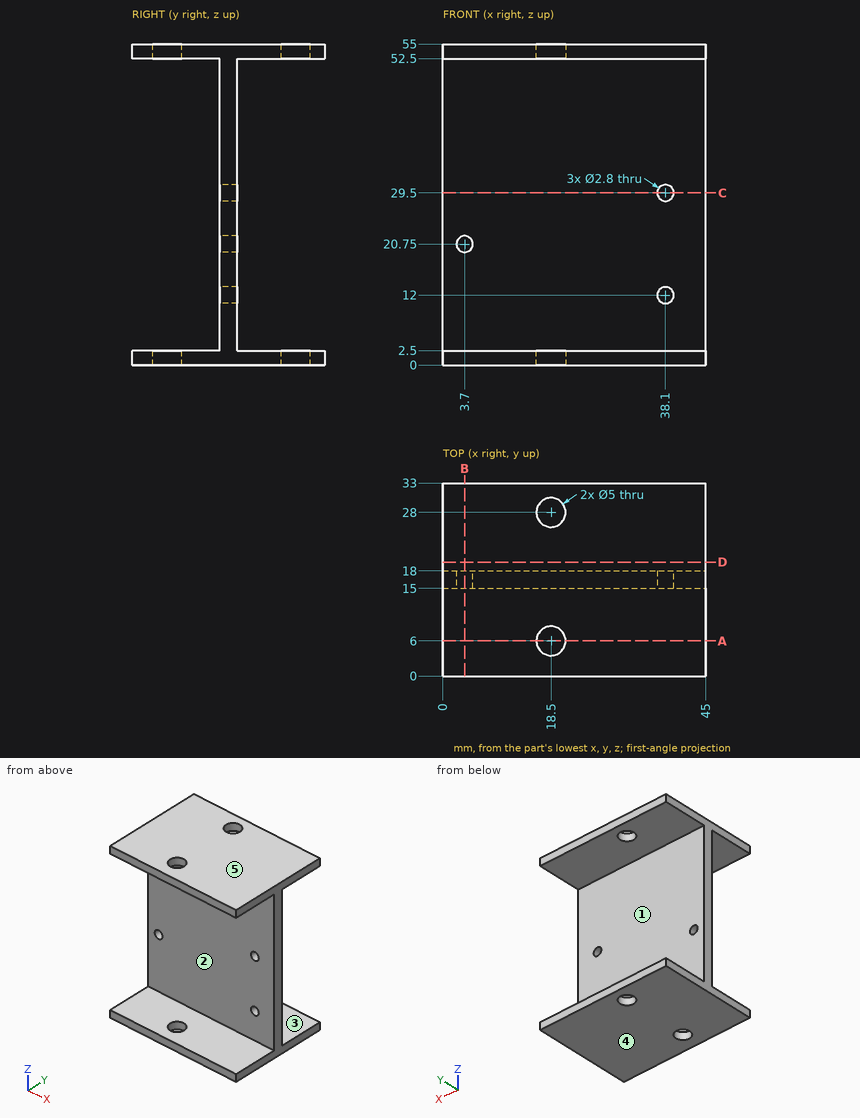
Verification items for this drawing (mm, ordinates from the low corner). A direction names the side the tool comes from. Give positions to 0.01 mm unless a question says otherwise; leave off trailing zeros. Write each loop counter-clockwise with the first axis right and the second up, starting at its lowest first coordinate (ties: lowest second). Pieces come first, ordered by that corner, then holes. Notation, with made-up numbers: (80.5, 72) -> (102.5, 72) arc R11 ccw to (102.5, 93) -> close; hole circle Ø2 at (20, -1.5). An arc over 180 degrees is marked (long way). Use CSV: the item, a comma, the result in double quotes. Start each with the question number.
Q1. Cross-section at A-A on y = 6. Enter the section's corners in (x, z).
Q2. Cross-section at B-B on x = 3.7. Enter the section's corners in (y, z).
Q3. Tool access check on the marked faces 1 and 2. Record the directions out of +Z, -Z, +X, -X, +Y, -Y that give a thin tool (end or side, any length) a straight path to the whole face; none if there is none.
Q4. Depth check by flat-ended pin: P1, Ø5, axis at x = 17, z = 31, coming from the +Y side; P2, Ø4.5, axis at x = 3.7, z = 20.75, coming from the -Y side. Enter the tip coordinate at first touch or a pass-through.
Q5. Cross-section at C-C on z = 29.5. Enter the section's corners in (x, y), and give its area (3 significant figures).
Q6. Release check for a two-part mould opening along Z. For the marked faces 3, 4 and 5 record: +Z half, -Z half, draft (parallel to the pull), parting line (faces both ways), or undercut.
Q7. Scan lines: line 1 along Y through (x, z) = (18.5, 54.55); line 2 along Z through (x, y) = (10, 5.5); line 3 along Z through (x, y) = (38.1, 15.95). Record each from-to range of solid material in increasing order.
Q8. Cross-section at D-D on y = 19.5. Enter the section's corners in (x, z).
Working result:
1,outline,"(0, 0) -> (16, 0) -> (16, 2.5) -> (0, 2.5) -> close; (0, 52.5) -> (16, 52.5) -> (16, 55) -> (0, 55) -> close; (21, 0) -> (45, 0) -> (45, 2.5) -> (21, 2.5) -> close; (21, 52.5) -> (45, 52.5) -> (45, 55) -> (21, 55) -> close"
2,outline,"(0, 0) -> (33, 0) -> (33, 2.5) -> (18, 2.5) -> (18, 19.35) -> (15, 19.35) -> (15, 2.5) -> (0, 2.5) -> close; (0, 52.5) -> (15, 52.5) -> (15, 22.15) -> (18, 22.15) -> (18, 52.5) -> (33, 52.5) -> (33, 55) -> (0, 55) -> close"
3,face 1,"+X, -X, +Y"
3,face 2,"+X, -X, -Y"
4,P1,"stops at y = 18"
4,P2,"stops at y = 15"
5,outline,"(0, 15) -> (36.7, 15) -> (36.7, 18) -> (0, 18) -> close; (39.5, 15) -> (45, 15) -> (45, 18) -> (39.5, 18) -> close"
5,area,"127 mm^2"
6,face 3,"undercut"
6,face 4,"-Z half"
6,face 5,"+Z half"
7,line 1,"y = 0 to 3.5, 8.5 to 25.5, 30.5 to 33"
7,line 2,"z = 0 to 2.5, 52.5 to 55"
7,line 3,"z = 0 to 10.6, 13.4 to 28.1, 30.9 to 55"
8,outline,"(0, 0) -> (45, 0) -> (45, 2.5) -> (0, 2.5) -> close; (0, 52.5) -> (45, 52.5) -> (45, 55) -> (0, 55) -> close"
